from build123d import *

# Parameters (mm, degrees)
ESTRUSIONE_ESTRUSIONE1_DEPTH = 6.5
SCHIZZO2_R                   = 1.7
TAGLIO_ESTRUSIONE1_DEPTH     = 6.5


with BuildPart() as part:
    # Schizzo1 → Estrusione-Estrusione1 (new body)
    with BuildSketch(Plane.XY):
        with BuildLine():
            Line((0, 4.2), (0, 12.2))
            Line((0, 12.2), (-2, 12.2))
            Line((-2, 12.2), (-2, 6.394528911))
            ThreePointArc((-2, 6.394528911), (-6.7, 0), (-2, -6.394528911))
            Line((-2, -6.394528911), (-2, -12.2))
            Line((-2, -12.2), (0, -12.2))
            Line((0, -12.2), (0, -4.2))
            ThreePointArc((0, -4.2), (-4.2, 0), (0, 4.2))
        make_face()
    extrude(amount=ESTRUSIONE_ESTRUSIONE1_DEPTH)

    # Schizzo2 → Taglio-Estrusione1 (cut)
    with BuildSketch(Plane.ZY.offset(2)):
        with Locations(Location((3.25, 9.297264456, 0), (0, 0, 270))):
            Circle(SCHIZZO2_R)
    taglio_estrusione1 = extrude(amount=-TAGLIO_ESTRUSIONE1_DEPTH, mode=Mode.SUBTRACT)

    # Specchia1: Taglio-Estrusione1 across plane
    add(taglio_estrusione1.mirror(Plane.ZX), mode=Mode.SUBTRACT)


solid = part.part
Can you work these out from the model? Positions are in its coordinate system, mm. A direction names the side the tool comes from. Coordinates: 2 decimals unless noted, no trailing zeros. Order: outer loops, then holes, each group sorted by start corner. A loop starts at its lowest first (then second) coordinate and runs counter-clockwise, first axis right, second up. Notation, with made-up numbers: (12, 55) - (19, 55) arc R28 ccw to (19, 73) - close; hole circle Ø5 at (-8, 23). An arc over 180 degrees is marked (long way). Answer as a JSON object with one key per item and string values. Group by question number.
Q1. Imagine slicing it at C-C (z = 1.25). Please give me the cut outline in (x, y).
Q2. Imagine slicing it at D-D (y = 8). Please give me the cut outline in (x, z).
Q3. Will these pins go through, and if not, where does the flat tip stop? P1, Ø3, axis at y = -8, z = 4.5, coming from the -X side; P2, Ø1.5, axis at y = 0, z = 2.5, coming from the +X side.
Q4. Imagine slicing it at A-A (z = 3.25). Please give me the cut outline in (x, y), and give its area (3 significant figures).
Q5. We'd pull the mould along Y, two halves only. Please class faces 4 (the face through (-5, 0, 6.5)), 5 (the face through (-1.014, -7.676, 3.761)), 6 (the face through (-1, 12.2, 3)), 7 (the face through (-1, -12.2, 3)): +Y half, -Y half, draft (parallel to the pull), parting line (faces both ways), or undercut.
Q6. I need wall thicknesses on line 1 (Y direction, x = -0.5, z = 3); line 2 (X direction, y = 8.5, z = 0.75); line 3 (Z direction, x = -1, y = 8.5). Which ranges of each line are inside material? Lowest first, please. Write a range as from..to.
Q7. Imagine slicing it at B-B (x = -0.5). Please give me the cut outline in (y, z), and give its area (3 significant figures).
Q8. On a 3-axis mill with a long thin cutter (end or side, diameter ignored), from which of +Z, -Z, +X, -X, +Y, -Y can I reach the whole of each face in a straight line? I mean faces 1 (the face through (0, 7, 3)), 2 (the face through (-2, -11.2, 3.2)), 3 (the face through (-2, 7, 3)). Say none if no direction works.
Determined:
{
 "1": {"outline": "(-2, -12.2) - (0, -12.2) - (0, -4.2) arc R4.2 cw to (0, 4.2) - (0, 12.2) - (-2, 12.2) - (-2, 6.39) arc R6.7 ccw to (-2, -6.39) - close"},
 "2": {"outline": "(-2, 0) - (0, 0) - (0, 2.15) - (-2, 2.15) - close; (-2, 4.35) - (0, 4.35) - (0, 6.5) - (-2, 6.5) - close"},
 "3": {"P1": "stops at x = -2", "P2": "stops at x = -4.13"},
 "4": {"outline": "(-2, -12.2) - (0, -12.2) - (0, -11) - (-2, -11) - close; (-2, -7.6) - (0, -7.6) - (0, -4.2) arc R4.2 cw to (0, 4.2) - (0, 7.6) - (-2, 7.6) - (-2, 6.39) arc R6.7 ccw to (-2, -6.39) - close; (-2, 11) - (0, 11) - (0, 12.2) - (-2, 12.2) - close", "area": "51.6 mm2"},
 "5": {"face 4": "draft", "face 5": "undercut", "face 6": "+Y half", "face 7": "-Y half"},
 "6": {"line 1": "y = -12.2..-10.98, -7.62..-4.17, 4.17..7.62, 10.98..12.2", "line 2": "x = -2..0", "line 3": "z = 0..1.75, 4.75..6.5"},
 "7": {"outline": "(-12.2, 0) - (-4.17, 0) - (-4.17, 6.5) - (-12.2, 6.5) - close; (4.17, 0) - (12.2, 0) - (12.2, 6.5) - (4.17, 6.5) - close; hole circle Ø3.4 at (-9.3, 3.25); hole circle Ø3.4 at (9.3, 3.25)", "area": "86.2 mm2"},
 "8": {"face 1": "+Z, -Z, +X, +Y, -Y", "face 2": "+Z, -Z, -X, -Y", "face 3": "+Z, -Z, -X, +Y"}
}
